```python
from build123d import *

# Parameters (mm, degrees)
SKETCH1_W           = 59.35
SKETCH1_H           = 59.35
BOSS_EXTRUDE1_DEPTH = 6
SKETCH2_R           = 1.5
CUT_EXTRUDE1_DEPTH  = 7
SKETCH7_W           = 55.9
SKETCH7_H           = 55.9
CUT_EXTRUDE3_DEPTH  = 1.85
CUT_EXTRUDE4_DEPTH  = 2.4
FILLET1_R           = 3
CHAMFER1_SIZE       = 0.25


with BuildPart() as part:
    # Sketch1 → Boss-Extrude1 (new body)
    with BuildSketch(Plane(origin=(0, 0, 0), x_dir=(1, 0, 0), z_dir=(0, 1, 0))):
        Rectangle(SKETCH1_W, SKETCH1_H)
    extrude(amount=BOSS_EXTRUDE1_DEPTH)

    # Sketch2 → Cut-Extrude1 (cut, through all)
    with BuildSketch(Plane(origin=(0, 6, 0), x_dir=(1, 0, 0), z_dir=(0, 1, 0))):
        with Locations((-24.5, 24.5)):
            Circle(SKETCH2_R)
        with Locations((24.5, 24.5)):
            Circle(SKETCH2_R)
        with Locations((-24.5, -24.5)):
            Circle(SKETCH2_R)
        with Locations((24.5, -24.5)):
            Circle(SKETCH2_R)
    extrude(amount=-CUT_EXTRUDE1_DEPTH, mode=Mode.SUBTRACT)

    # Sketch7 → Cut-Extrude3 (cut)
    with BuildSketch(Plane(origin=(0, 6, 0), x_dir=(1, 0, 0), z_dir=(0, 1, 0))):
        Rectangle(SKETCH7_W, SKETCH7_H)
    extrude(amount=-CUT_EXTRUDE3_DEPTH, mode=Mode.SUBTRACT)

    # Sketch8 → Cut-Extrude4 (cut)
    with BuildSketch(Plane(origin=(0, 4.15, 0), x_dir=(1, 0, 0), z_dir=(0, 1, 0))):
        Polygon((-27.95, 21.45), (-21.45, 21.45), (-21.45, 27.95), (21.45, 27.95), (21.45, 21.45), (27.95, 21.45), (27.95, -21.45), (21.45, -21.45), (21.45, -27.95), (-21.45, -27.95), (-21.45, -21.45), (-27.95, -21.45), align=None)
    extrude(amount=-CUT_EXTRUDE4_DEPTH, mode=Mode.SUBTRACT)

    # Fillet1
    fillet1_edges = [part.edges().sort_by_distance(p)[0] for p in [
        (-21.45, 2.95, -21.45),
        (21.45, 2.95, -21.45),
        (21.45, 2.95, 21.45),
        (-21.45, 2.95, 21.45),
        (-29.675, 3, 29.675),
        (-29.675, 3, -29.675),
        (29.675, 3, -29.675),
        (29.675, 3, 29.675),
    ]]
    fillet(fillet1_edges, radius=FILLET1_R)

    # Chamfer1
    chamfer1_edges = [part.edges().sort_by_distance(p)[0] for p in [
        (-26, 4.15, -24.5),
        (23, 4.15, 24.5),
        (-26, 4.15, 24.5),
        (23, 4.15, -24.5),
    ]]
    chamfer(chamfer1_edges, length=CHAMFER1_SIZE)


solid = part.part
```
Geometry check sheet. Reference: the model listing, model coordinates, mm. A direction names the side the tool comes from. Coordinates: 2 decimals unless noted, no trailing zeros. Write each loop counter-clockwise with the first axis right and the second up, starting at its lowest first coordinate (ties: lowest second). Pieces come first, ordered by that corner, then holes. Notation, with made-up numbers: (63.25, -22) -> (91.25, -22) arc R8 ccw to (91.25, -14) -> close; hole circle Ø7 at (-18, 59). An arc over 180 degrees is marked (long way). Use CSV: the item, a comma, the result in double quotes. Start each with the question number.
Item 1: Cross-section at B-B, the plane x = -7. Record the cut outline in (y, z) (3 decimals), plus the area to 3 significant figures.
Item 2: Set-up check for faces 1 (the flat face through (21.45, 3, -26)), 2 (the flat face through (0, 0, 0)): record each of +Z, -Z, +X, -X, +Y, -Y from which the full face is reachable in a straight line by a thin tool's end or side.
Item 3: Mould release check, pull along X, two halves, no side actions. Record for faces 3 (the cylindrical face through (28.77, 3.04, 28.82)), 4 (the flat face through (-27.95, 4, 0)), 5 (the flat face through (-2.3, 6, 28.4)): released by +X, released by -X, zero draft, split by the parting line, or undercut.
Item 4: Depth check by flat-ended pin: pin 1 Ø5 at (x, z) = (-24, -26) entering from +Y; pin 2 Ø7 at (x, z) = (24, -24) entering from +Y; pin 3 Ø5 at (x, z) = (22.5, -19) entering from +Y. Enter the tip coordinate at first touch or a pass-through.
Item 5: Thickness scan on line 1 (X direction, y = 0.95, z = 24.5) (3 decimals); line 2 (Z direction, x = -24.5, y = 2.45) (3 decimals); line 3 (X direction, y = 4.7, z = 26) (3 decimals). Record the ranges inside material, lowest first.
Item 6: Cross-section at A-A, the plane z = -20.5. Record the cut outline in (x, y) (3 decimals), plus the area to 3 significant figures.
Answers:
1,outline,"(0, -29.675) -> (6, -29.675) -> (6, -27.95) -> (1.75, -27.95) -> (1.75, 27.95) -> (6, 27.95) -> (6, 29.675) -> (0, 29.675) -> close"
1,area,"119 mm^2"
2,face 1,"+Y"
2,face 2,"+Z, -Z, +X, -X, -Y"
3,face 3,"released by +X"
3,face 4,"undercut"
3,face 5,"zero draft"
4,pin 1,"y = 6"
4,pin 2,"y = 4.15"
4,pin 3,"y = 1.75"
5,line 1,"-29.675 to -26, -23 to 23, 26 to 29.675"
5,line 2,"-29.675 to -26, -23 to -21.45, 21.45 to 23, 26 to 29.675"
5,line 3,"-29.675 to -27.95, 27.95 to 29.675"
6,outline,"(-29.675, 0) -> (29.675, 0) -> (29.675, 6) -> (27.95, 6) -> (27.95, 1.75) -> (-27.95, 1.75) -> (-27.95, 6) -> (-29.675, 6) -> close"
6,area,"119 mm^2"
